from build123d import *

# Parameters (mm, degrees)
F0_W     = 127
F0_H     = 50.8
F1_DEPTH = 152.4
F2_W     = 76.2
F2_H     = 50.8
F3_DEPTH = 101.6
F5_DEPTH = 101.6
F6_W     = 127
F6_H     = 50.8
F7_DEPTH = 76.2


with BuildPart() as f1:
    # F0 (on Front) → F1 (new body)
    with BuildSketch(Plane.XZ):
        with Locations((-12.272136, -61.733169)):
            Rectangle(F0_W, F0_H)
    extrude(amount=F1_DEPTH)

    # F2 (on face) → F3 (join)
    with BuildSketch(Plane.XY.offset(-36.333169)):
        with Locations((-37.672136, -25.4)):
            Rectangle(F2_W, F2_H)
    extrude(amount=F3_DEPTH)

    # F4 (on face) → F5 (join)
    with BuildSketch(Plane.XY.offset(-36.333169)):
        Polygon((51.227864, -127), (51.227864, 0), (0.427864, 0), (0.427864, -50.8), (0, -50.8), (0, -127), align=None)
    extrude(amount=F5_DEPTH)

    # F6 (on face) → F7 (join)
    with BuildSketch(Plane(origin=(0, 0, 0), x_dir=(-1, 0, 0), z_dir=(0, 1, 0))):
        with Locations((12.272136, 39.866831)):
            Rectangle(F6_W, F6_H)
    extrude(amount=F7_DEPTH)


solid = f1.part
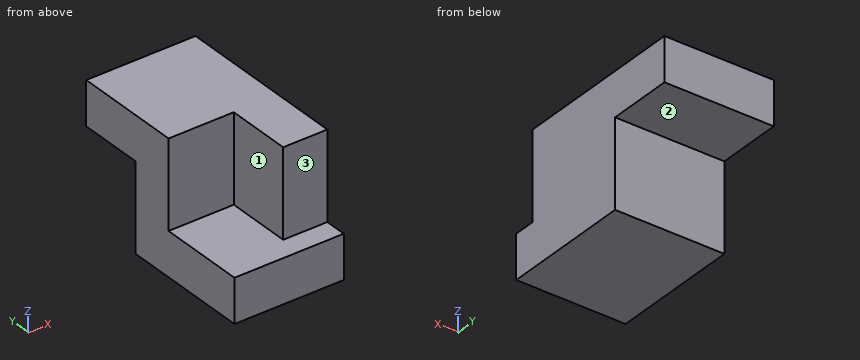
Could you check a few things on this model? Use its own coordinates, in mm. Face numbers are marked on the shaded views. A direction names the side the tool comes from. Coordinates: 2 decimals unless noted, no trailing zeros. Loops run counter-clockwise (first coordinate to the right, second up) from the corner with the lowest first, then second, coordinate; pieces in that order, holes last. Notation, with made-up numbers: (-38.5, -8.75) -> (-7.5, -8.75) arc R11 cw to (-7.5, 0.25) -> close; hole circle Ø6 at (53.25, 46.25). An arc over 180 degrees is marked (long way). Answer in a Markdown table with one row per item.
(1) Will these pins go through, and if not, where does the flat tip stop? pin 1 Ø2 at (x, y) = (-33, -123.5) entering from +Z; pin 2 Ø12 at (x, z) = (-38, -70.5) entering from +Y; pin 3 Ø1.5 at (x, z) = (6.5, 42.5) entering from -Y.
Results found:
| item | result |
|---|---|
| pin 1 | stops at z = -36.33 |
| pin 2 | stops at y = 0 |
| pin 3 | stops at y = -127 |
(2) Imagine slicing it at C-C (y = -124). List the corners of the cut face in (x, z) for me.
Results found:
| item | result |
|---|---|
| outline | (-75.77, -87.13) -> (51.23, -87.13) -> (51.23, 65.27) -> (0, 65.27) -> (0, -36.33) -> (-75.77, -36.33) -> close |
(3) Imagine slicing it at B-B (z = -32.5). List the corners of the cut face in (x, y) for me, plus the area to 3 significant figures.
Results found:
| item | result |
|---|---|
| outline | (-75.77, -50.8) -> (0, -50.8) -> (0, -127) -> (51.23, -127) -> (51.23, 0) -> (-75.77, 0) -> close |
| area | 10,400 mm^2 |
(4) If I drill on probe 1 along Y at (x, z) = (21.5, -60); probe 2 along Y at (x, z) = (34, 16); probe 3 along X at (y, z) = (-76, -31), over which ranges is the centre line in solid material (lowest first)?
Results found:
| item | result |
|---|---|
| probe 1 | y = -152.4 to 0 |
| probe 2 | y = -127 to 76.2 |
| probe 3 | x = 0 to 51.23 |
(5) For the marked faces 1, 2 and 3, which set-ups out of +Z, -Z, +X, -X, +Y, -Y let a thin tool reach every point of the face, with its end or its side?
Results found:
| item | result |
|---|---|
| face 1 | +Z, -X, -Y |
| face 2 | -Z, +X, -X, +Y |
| face 3 | +Z, +X, -X, -Y |
(6) Imagine slicing it at D-D (x = -60.5). List the corners of the cut face in (y, z) for me, plus the area to 3 significant figures.
Results found:
| item | result |
|---|---|
| outline | (-152.4, -87.13) -> (0, -87.13) -> (0, 14.47) -> (76.2, 14.47) -> (76.2, 65.27) -> (-50.8, 65.27) -> (-50.8, -36.33) -> (-152.4, -36.33) -> close |
| area | 16,800 mm^2 |
(7) Imagine slicing it at A-A (x = 41). List the corners of the cut face in (y, z) for me, plus the area to 3 significant figures.
Results found:
| item | result |
|---|---|
| outline | (-152.4, -87.13) -> (0, -87.13) -> (0, 14.47) -> (76.2, 14.47) -> (76.2, 65.27) -> (-127, 65.27) -> (-127, -36.33) -> (-152.4, -36.33) -> close |
| area | 24,500 mm^2 |
